Part model, mm, in its own coordinate system. A direction names the side the tool comes from. Round coordinates to 2 decimals unless told otherwise and drop trailing zeros. Loops run counter-clockwise (first coordinate to the right, second up) from the corner with the lowest first, then second, coordinate; pieces in that order, holes last.
1) Band-saw the part on C-C, the plane z = 7. Write the cut outline in (x, y).
2) Drop flat-ended pins along their axis: P1, Ø3, axis at x = -11.5, z = -7, coming from the +Y side; P2, Ø2.5, axis at x = 12.12, z = -7, coming from the +Y side. Give the stop position or say it passes through.
3) Band-saw the part on A-A, the plane z = 0. Write the cut outline in (x, y).
4) Mould opens along X. For faces 1 (the flat face through (-10, 0, -7)), 2 (the cylindrical face through (-19.72, 0.04, 19.65)), 3 (the flat face through (0, 0, 21.15)) say: +X half, -X half, draft (parallel to the pull), parting line (faces both ways), or undercut.
5) 3-axis set-ups, long thin cutter, end or side, ignore diameter. For faces 4 (the cylindrical face through (-9.263, 1.521, 6.099)), 5 (the flat face through (-10, 3, 0)): which of +Z, -Z, +X, -X, +Y, -Y reach the whole face in a straight line?
6) Band-saw the part on D-D, the plane x = 5.5. Write the cut outline in (y, z).
7) Probe line 1 (Z direction, x = 15.5, y = -1.2); line 2 (Z direction, x = 0, y = 0.8); line 3 (Z direction, x = 14, y = -0.9). List the from-to ranges inside material, lowest first.
8) Band-saw the part on B-B, the plane x = -1. Write the cut outline in (y, z), then the cut area to 3 significant figures.
from build123d import *

# Parameters (mm, degrees)
SKETCH1_W           = 42.3
SKETCH1_H           = 42.3
BOSS_EXTRUDE1_DEPTH = 3
FILLET1_R           = 5
SKETCH2_R           = 1.75
CUT_EXTRUDE1_DEPTH  = 7
SKETCH4_R           = 9.5
CUT_EXTRUDE3_DEPTH  = 7
SKETCH5_R           = 1.55
CUT_EXTRUDE4_DEPTH  = 7
SKETCH6_R           = 3
CUT_EXTRUDE5_DEPTH  = 3
CIRPATTERN1_COUNT   = 6


with BuildPart() as part:
    # Sketch1 → Boss-Extrude1 (new body, symmetric)
    with BuildSketch(Plane(origin=(0, 0, 0), x_dir=(1, 0, 0), z_dir=(0, 1, 0))):
        Rectangle(SKETCH1_W, SKETCH1_H)
    extrude(amount=BOSS_EXTRUDE1_DEPTH, both=True)

    # Fillet1
    fillet1_edges = [part.edges().sort_by_distance(p)[0] for p in [
        (21.15, 0, 21.15),
        (-21.15, 0, 21.15),
        (-21.15, 0, -21.15),
        (21.15, 0, -21.15),
    ]]
    fillet(fillet1_edges, radius=FILLET1_R)

    # Sketch2 → Cut-Extrude1 (cut, through all)
    with BuildSketch(Plane.XZ.offset(3)):
        with Locations((-15.5, 15.5)):
            Circle(SKETCH2_R)
        with Locations((15.5, 15.5)):
            Circle(SKETCH2_R)
        with Locations((15.5, -15.5)):
            Circle(SKETCH2_R)
        with Locations((-15.5, -15.5)):
            Circle(SKETCH2_R)
    extrude(amount=-CUT_EXTRUDE1_DEPTH, mode=Mode.SUBTRACT)

    # Sketch4 → Cut-Extrude3 (cut, through all)
    with BuildSketch(Plane.XZ.offset(3)):
        Circle(SKETCH4_R)
    extrude(amount=-CUT_EXTRUDE3_DEPTH, mode=Mode.SUBTRACT)

    # Sketch5 → Cut-Extrude4 (cut, through all)
    with BuildSketch(Plane(origin=(0, 3, 0), x_dir=(1, 0, 0), z_dir=(0, 1, 0))):
        with Locations((0, 14)):
            Circle(SKETCH5_R)
    cut_extrude4 = extrude(amount=-CUT_EXTRUDE4_DEPTH, mode=Mode.SUBTRACT)

    # Sketch6 → Cut-Extrude5 (cut)
    with BuildSketch(Plane(origin=(0, 3, 0), x_dir=(1, 0, 0), z_dir=(0, 1, 0))):
        with Locations((0, 14)):
            Circle(SKETCH6_R)
    cut_extrude5 = extrude(amount=-CUT_EXTRUDE5_DEPTH, mode=Mode.SUBTRACT)

    # CirPattern1: Cut-Extrude4, Cut-Extrude5 ×6 about axis
    cirpattern1_axis = Axis((0, 0, 0), (0, 1, 0))
    for i in range(1, CIRPATTERN1_COUNT):
        add(cut_extrude4.rotate(cirpattern1_axis, i * 360 / CIRPATTERN1_COUNT), mode=Mode.SUBTRACT)
        add(cut_extrude5.rotate(cirpattern1_axis, i * 360 / CIRPATTERN1_COUNT), mode=Mode.SUBTRACT)


solid = part.part
Reported:
1. outline: (-21.15, -3) - (-13.67, -3) - (-13.67, 0) - (-15.12, 0) - (-15.12, 3) - (-21.15, 3) - close; (-10.57, -3) - (-6.42, -3) - (-6.42, 3) - (-9.12, 3) - (-9.12, 0) - (-10.57, 0) - close; (6.42, -3) - (10.57, -3) - (10.57, 0) - (9.12, 0) - (9.12, 3) - (6.42, 3) - close; (13.67, -3) - (21.15, -3) - (21.15, 3) - (15.12, 3) - (15.12, 0) - (13.67, 0) - close
2. P1: stops at y = 0
2. P2: passes through
3. outline: (-21.15, -3) - (-9.5, -3) - (-9.5, 3) - (-21.15, 3) - close; (9.5, -3) - (21.15, -3) - (21.15, 3) - (9.5, 3) - close
4. face 1: undercut
4. face 2: -X half
4. face 3: draft
5. face 4: +Y
5. face 5: +Z, -Z, +X, -X, +Y
6. outline: (-3, -21.15) - (3, -21.15) - (3, -7.75) - (-3, -7.75) - close; (-3, 7.75) - (3, 7.75) - (3, 21.15) - (-3, 21.15) - close
7. line 1: z = -21.15 to -17.25, -13.75 to 13.75, 17.25 to 21.15
7. line 2: z = -21.15 to -17, -11 to -9.5, 9.5 to 11, 17 to 21.15
7. line 3: z = -21.15 to -16.4, -14.6 to 14.6, 16.4 to 21.15
8. outline: (-3, -21.15) - (3, -21.15) - (3, -16.83) - (0, -16.83) - (0, -15.18) - (-3, -15.18) - close; (-3, -12.82) - (0, -12.82) - (0, -11.17) - (3, -11.17) - (3, -9.45) - (-3, -9.45) - close; (-3, 9.45) - (3, 9.45) - (3, 11.17) - (0, 11.17) - (0, 12.82) - (-3, 12.82) - close; (-3, 15.18) - (0, 15.18) - (0, 16.83) - (3, 16.83) - (3, 21.15) - (-3, 21.15) - close
8. area: 92.3 mm2
